```python
from build123d import *

# Parameters (mm, degrees)
SKETCH1_W           = 69.85
SKETCH1_H           = 6.35
BOSS_EXTRUDE1_DEPTH = 120.65
CUT_EXTRUDE1_DEPTH  = 140.555607197
SKETCH3_W           = 5.08
SKETCH3_H           = 120.65
CUT_EXTRUDE2_DEPTH  = 42.164
SKETCH4_W           = 2.54
SKETCH4_H           = 22.86
CUT_EXTRUDE3_DEPTH  = 6.35
SKETCH5_W           = 11.5316
SKETCH5_H           = 12.7
BOSS_EXTRUDE2_DEPTH = 6.35
SKETCH6_R           = 1.778
CUT_EXTRUDE4_DEPTH  = 6.35


with BuildPart() as part:
    # Sketch1 → Boss-Extrude1 (new body)
    with BuildSketch(Plane.XY):
        with Locations((34.925, 3.175)):
            Rectangle(SKETCH1_W, SKETCH1_H)
    extrude(amount=BOSS_EXTRUDE1_DEPTH)

    # Sketch2 → Cut-Extrude1 (cut, through all)
    with BuildSketch(Plane(origin=(0, 6.35, 0), x_dir=(1, 0, 0), z_dir=(0, 1, 0))):
        Polygon((35.923749516, 0), (35.923749516, -37.802999389), (69.85, -55.962276793), (69.85, 0), align=None)
    extrude(amount=-CUT_EXTRUDE1_DEPTH, mode=Mode.SUBTRACT)

    # Sketch3 → Cut-Extrude2 (cut)
    with BuildSketch(Plane.XZ):
        Polygon((19.1516, 120.65), (19.1516, 0), (35.923749516, 0), (35.923749516, 37.802999389), (69.85, 55.962276793), (69.85, 120.65), align=None)
        with Locations((2.54, 60.325)):
            Rectangle(SKETCH3_W, SKETCH3_H)
    extrude(amount=-CUT_EXTRUDE2_DEPTH, mode=Mode.SUBTRACT)

    # Sketch4 → Cut-Extrude3 (cut)
    with BuildSketch(Plane.XZ):
        with Locations((6.35, 77.47)):
            Rectangle(SKETCH4_W, SKETCH4_H)
        with Locations((17.8816, -1.27)):
            Rectangle(SKETCH4_W, SKETCH4_H)
    extrude(amount=-CUT_EXTRUDE3_DEPTH, mode=Mode.SUBTRACT)

    # Sketch5 → Boss-Extrude2 (add)
    with BuildSketch(Plane.XZ):
        with Locations((10.8458, -6.35)):
            Rectangle(SKETCH5_W, SKETCH5_H)
    extrude(amount=-BOSS_EXTRUDE2_DEPTH)

    # Sketch6 → Cut-Extrude4 (cut)
    with BuildSketch(Plane.XZ):
        with Locations(Location((12.1666, 88.9, 0), (0, 0, 270))):
            Circle(SKETCH6_R)
        with Locations(Location((12.1666, 68.834, 0), (0, 0, 270))):
            Circle(SKETCH6_R)
        Circle(SKETCH6_R)
        with Locations(Location((12.1666, 48.768, 0), (0, 0, 270))):
            Circle(SKETCH6_R)
        with Locations(Location((12.1666, 28.702, 0), (0, 0, 270))):
            Circle(SKETCH6_R)
        with Locations(Location((12.1666, 8.636, 0), (0, 0, 270))):
            Circle(SKETCH6_R)
    extrude(amount=-CUT_EXTRUDE4_DEPTH, mode=Mode.SUBTRACT)


solid = part.part
```
Part model, mm, in its own coordinate system. A direction names the side the tool comes from. Coordinates: 2 decimals unless noted, no trailing zeros. Order: outer loops, then holes, each group sorted by start corner. A loop starts at its lowest first (then second) coordinate and runs counter-clockwise, first axis right, second up. Notation, with made-up numbers: (-30.75, 73.5) - (28.25, 73.5) arc R17 cw to (28.25, 81.5) - close; hole circle Ø7 at (34.25, -26). An arc over 180 degrees is marked (long way). Return JSON: item names as keys, results as strings. Group by question number.
Item 1: Which spindle directions (+Z, -Z, +X, -X, +Y, -Y) get a long thin tool onto all of the face, cutting with end or side? Do faces 1 (the face through (18, 3, 10.16)), 2 (the face through (6, 3, 66.04)), 3 (the face through (12, 6.35, 55)). Say none if no direction does.
Item 2: Drill centre lines: probe 1 along Z at (x, y) = (12.25, 2.75); probe 2 along Z at (x, y) = (6, 3.75); probe 3 along Z at (x, y) = (12.5, 4.5). Where is each one in solid material? Low to high. Write a range as from..to.
Item 3: Cut at B-B (x = 17.75). List the corners of the cut face in (y, z).
Item 4: Cut at A-A (y = 2.25). List the corners of the cut face in (x, z).
Item 5: Cut at C-C (z = 77.5). List the corners of the cut face in (x, y).
Item 6: Pull direction X, two halves, no side cores. Call faces 4 (the face through (16.612, 3, -1)), 5 (the face through (12, 3, 120.65)), 6 (the face through (12.245, 3.131, 90.676)), 7 (the face through (11.486, 3.131, 47.126)): pulls with the +X half, pulls with the -X half, needs draft (parallel to the pull), parting line crosses it, or undercut.
Check values:
{
 "1": {"face 1": "-Z, +X, +Y, -Y", "face 2": "-X, +Y, -Y", "face 3": "+Z, -Z, +X, -X, +Y"},
 "2": {"probe 1": "z = -12.7..6.86, 10.41..26.93, 30.48..46.99, 50.54..67.06, 70.61..87.12, 90.68..120.65", "probe 2": "z = -12.7..66.04, 88.9..120.65", "probe 3": "z = -12.7..6.89, 10.38..26.96, 30.45..47.02, 50.51..67.09, 70.58..87.15, 90.65..120.65"},
 "3": {"outline": "(0, 10.16) - (6.35, 10.16) - (6.35, 120.65) - (0, 120.65) - close"},
 "4": {"outline": "(5.08, -12.7) - (16.61, -12.7) - (16.61, 10.16) - (19.15, 10.16) - (19.15, 120.65) - (5.08, 120.65) - (5.08, 88.9) - (7.62, 88.9) - (7.62, 66.04) - (5.08, 66.04) - close; hole circle Ø3.56 at (12.17, 8.64); hole circle Ø3.56 at (12.17, 28.7); hole circle Ø3.56 at (12.17, 48.77); hole circle Ø3.56 at (12.17, 68.83); hole circle Ø3.56 at (12.17, 88.9)"},
 "5": {"outline": "(7.62, 0) - (19.15, 0) - (19.15, 6.35) - (7.62, 6.35) - close"},
 "6": {"face 4": "pulls with the +X half", "face 5": "needs draft", "face 6": "undercut", "face 7": "undercut"}
}
